```python
from build123d import *

# Parameters (mm, degrees)
SKETCH1_W           = 100
SKETCH1_H           = 60
BOSS_EXTRUDE1_DEPTH = 12
FILLET1_R           = 5
SKETCH2_R           = 15
BOSS_EXTRUDE2_DEPTH = 20
CHAMFER1_SIZE       = 1
SKETCH3_R           = 8
CUT_EXTRUDE2_DEPTH  = 67.513156593
SKETCH4_R           = 5
CUT_EXTRUDE4_DEPTH  = 3
SKETCH5_R           = 3
CUT_EXTRUDE6_DEPTH  = 62.64414003
SKETCH6_W           = 30
SKETCH6_H           = 8
CUT_EXTRUDE8_DEPTH  = 3
SKETCH7_R           = 1.5
CUT_EXTRUDE10_DEPTH = 8
CIRPATTERN1_COUNT   = 6
RIB2_REACH          = 68.513
SKETCH8_2_WALL_W    = 153.794637566
SKETCH8_2_WALL_H    = 6


with BuildPart() as part:
    # Sketch1 → Boss-Extrude1 (new body)
    with BuildSketch(Plane.XY):
        Rectangle(SKETCH1_W, SKETCH1_H)
    extrude(amount=BOSS_EXTRUDE1_DEPTH)

    # Fillet1
    fillet1_edges = [part.edges().sort_by_distance(p)[0] for p in [
        (-50, 30, 6),
        (50, 30, 6),
        (50, -30, 6),
        (-50, -30, 6),
    ]]
    fillet(fillet1_edges, radius=FILLET1_R)

    # Sketch2 → Boss-Extrude2 (add)
    with BuildSketch(Plane.XY.offset(12)):
        Circle(SKETCH2_R)
    extrude(amount=BOSS_EXTRUDE2_DEPTH)

    # Chamfer1
    chamfer1_edges = [part.edges().sort_by_distance(p)[0] for p in [
        (-15, 0, 32),
    ]]
    chamfer(chamfer1_edges, length=CHAMFER1_SIZE)

    # Sketch3 → Cut-Extrude2 (cut, through all)
    with BuildSketch(Plane.XY.offset(32)):
        Circle(SKETCH3_R)
    extrude(amount=-CUT_EXTRUDE2_DEPTH, mode=Mode.SUBTRACT)

    # Sketch4 → Cut-Extrude4 (cut)
    with BuildSketch(Plane.XY.offset(12)):
        with Locations((-40, -20)):
            Circle(SKETCH4_R)
        with Locations((-40, 20)):
            Circle(SKETCH4_R)
        with Locations((40, -20)):
            Circle(SKETCH4_R)
        with Locations((40, 20)):
            Circle(SKETCH4_R)
    extrude(amount=-CUT_EXTRUDE4_DEPTH, mode=Mode.SUBTRACT)

    # Sketch5 → Cut-Extrude6 (cut, through all)
    with BuildSketch(Plane.XY.offset(12)):
        with Locations((-40, -20)):
            Circle(SKETCH5_R)
        with Locations((-40, 20)):
            Circle(SKETCH5_R)
        with Locations((40, -20)):
            Circle(SKETCH5_R)
        with Locations((40, 20)):
            Circle(SKETCH5_R)
    extrude(amount=-CUT_EXTRUDE6_DEPTH, mode=Mode.SUBTRACT)

    # Sketch6 → Cut-Extrude8 (cut)
    with BuildSketch(Plane.XY.offset(12)):
        with Locations((0, -22.5)):
            Rectangle(SKETCH6_W, SKETCH6_H)
    extrude(amount=-CUT_EXTRUDE8_DEPTH, mode=Mode.SUBTRACT)

    # Sketch7 → Cut-Extrude10 (cut)
    with BuildSketch(Plane.XY.offset(32)):
        with Locations((12, 0)):
            Circle(SKETCH7_R)
    cut_extrude10 = extrude(amount=-CUT_EXTRUDE10_DEPTH, mode=Mode.SUBTRACT)

    # CirPattern1: Cut-Extrude10 ×6 about axis
    cirpattern1_axis = Axis((0, 0, 0), (0, 0, 1))
    for i in range(1, CIRPATTERN1_COUNT):
        add(cut_extrude10.rotate(cirpattern1_axis, i * 360 / CIRPATTERN1_COUNT), mode=Mode.SUBTRACT)

    # Sketch8_2 wall → Rib2 (add, up to next)
    with BuildSketch(Plane(origin=(0, 20.75, 19), x_dir=(0, -0.666015769309, 0.745937661626), z_dir=(0, -0.745937661626, -0.666015769309)), mode=Mode.PRIVATE) as rib2_sk1:
        Rectangle(SKETCH8_2_WALL_W, SKETCH8_2_WALL_H)
    rib2_tool1 = extrude(rib2_sk1.sketch, amount=RIB2_REACH, mode=Mode.PRIVATE) - part.part
    add(rib2_tool1.solids().sort_by_distance((0, 20.75, 19))[0])


solid = part.part
```
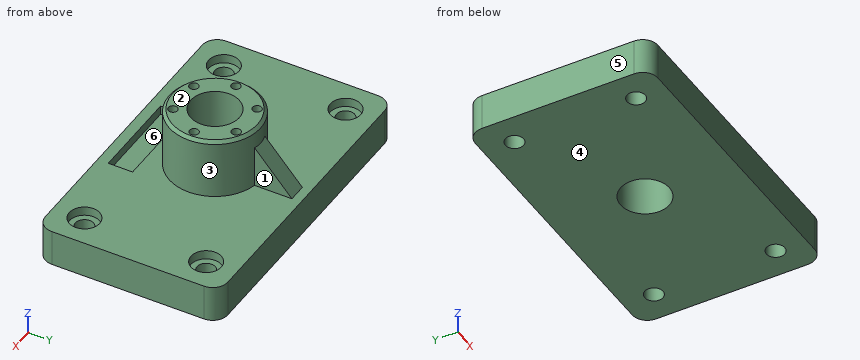
Can you work these out from the model? Positions are in its coordinate system, mm. Face numbers are marked on the shaded views. A direction names the side the tool comes from. Give positions to 0.01 mm unless a question says otherwise; leave off trailing zeros. Loops run counter-clockwise (first coordinate to the right, second up) from the corner with the lowest first, then second, coordinate; pieces in that order, holes last. Notation, with made-up numbers: M 3.25,-30.5 L 17.25,-30.5 A14 ccw 17.25,-17.5 Z; hole C -7.75,75.5 d8. An arc over 180 degrees is marked long. One line per item, written item: value.
(1) Which directions (+Z, -Z, +X, -X, +Y, -Y) give clear straight access to the entire face, cutting with the end or side of a thin tool? Please do the marked faces 1, 2 and 3.
Returned:
face 1: +Z, +X, +Y
face 2: +Z, +X, -X, +Y, -Y
face 3: +Z
(2) Suppose I cut it at B-B on y = -20. List the corners of the cut face in (x, z) for me, plus the area to 3 significant figures.
Returned:
outline: M -50,0 L -43,0 L -43,9 L -45,9 L -45,12 L -50,12 Z; M -37,0 L 37,0 L 37,9 L 35,9 L 35,12 L 15,12 L 15,9 L -15,9 L -15,12 L -35,12 L -35,9 L -37,9 Z; M 43,0 L 50,0 L 50,12 L 45,12 L 45,9 L 43,9 Z
area: 942 mm^2
(3) We'd pull the mould along X, two halves only. Please class the marked faces 4, 5 and 6: released by +X, released by -X, zero draft, split by the parting line, or undercut.
Returned:
face 4: zero draft
face 5: released by -X
face 6: undercut
(4) I need wall thicknesses on line 1 (Y direction, x = -40, z = 2); line 2 (X direction, y = -22, z = 11.5); line 3 (X direction, y = 17.5, z = 1.5). Which ranges of each line are inside material? Lowest first, please.
Returned:
line 1: -30 to -23, -17 to 17, 23 to 30
line 2: -50 to -44.58, -35.42 to -15, 15 to 35.42, 44.58 to 50
line 3: -50 to -41.66, -38.34 to 38.34, 41.66 to 50
(5) Will these pins go through, and if not, where does the flat tip stop? pin 1 (6 mm diameter, centred on y = 21.5, z = 16, fed in from -X); pin 2 (13 mm diameter, centred on x = -40, y = 20, fed in from +Z); pin 3 (8 mm diameter, centred on x = 39.5, y = -19.5, fed in from +Z).
Returned:
pin 1: x = -3
pin 2: z = 12
pin 3: z = 9
(6) Suppose I cut it at D-D on z = 2. List the corners of the cut face in (x, y) for me.
Returned:
outline: M -50,-25 A5 ccw -45,-30 L 45,-30 A5 ccw 50,-25 L 50,25 A5 ccw 45,30 L -45,30 A5 ccw -50,25 Z; hole C -40,-20 d6; hole C -40,20 d6; hole C 0,0 d16; hole C 40,-20 d6; hole C 40,20 d6
(7) Suppose I cut it at C-C on x = 40. List the corners of the cut face in (y, z) for me.
Returned:
outline: M -30,0 L -23,0 L -23,9 L -25,9 L -25,12 L -30,12 Z; M -17,0 L 17,0 L 17,9 L 15,9 L 15,12 L -15,12 L -15,9 L -17,9 Z; M 23,0 L 30,0 L 30,12 L 25,12 L 25,9 L 23,9 Z
(8) Suppose I cut it at A-A on z = 10. List the corners of the cut face in (x, y) for me, plus the area to 3 significant figures.
Returned:
outline: M -50,-25 A5 ccw -45,-30 L 45,-30 A5 ccw 50,-25 L 50,25 A5 ccw 45,30 L -45,30 A5 ccw -50,25 Z; hole C -40,-20 d10; hole C -40,20 d10; hole M -15,-26.5 L 15,-26.5 L 15,-18.5 L -15,-18.5 Z; hole C 0,0 d16; hole C 40,-20 d10; hole C 40,20 d10
area: 5,220 mm^2
